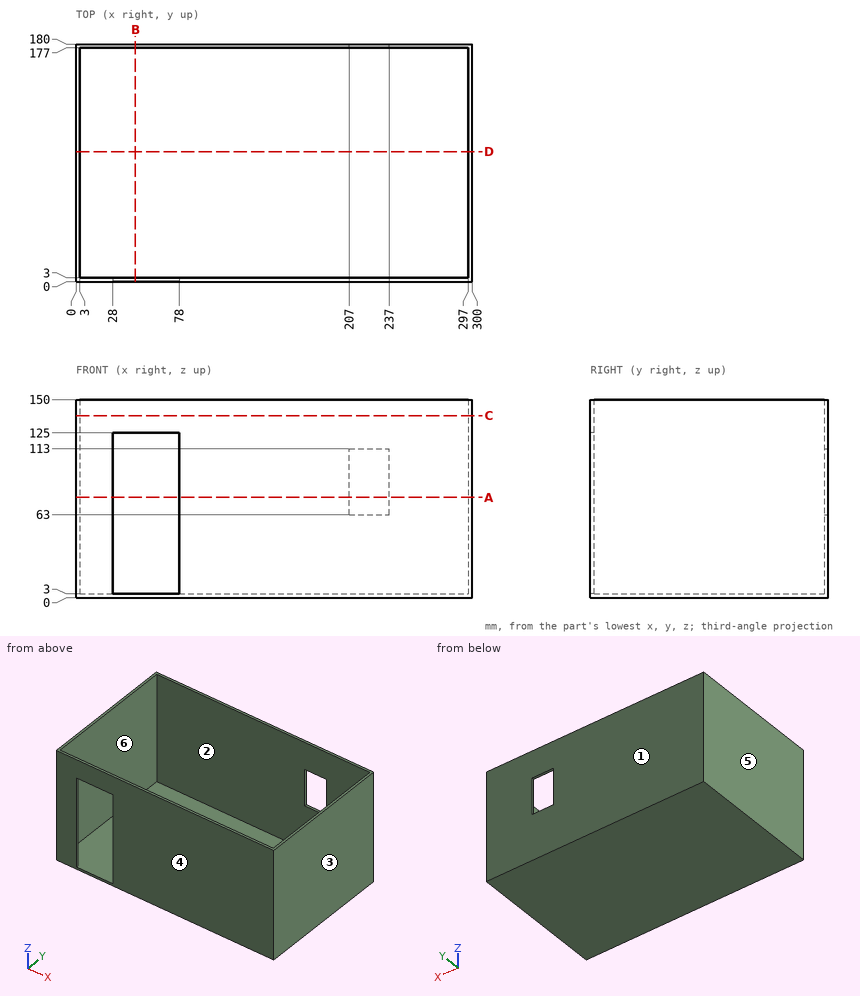
Could you check a few things on this drawing? It's one solid part, dimensions in mm from its lowest x, y, z. A direction names the side the tool comes from. Give positions to 0.01 mm unless a question says otherwise; leave off trailing zeros. Write each loop counter-clockwise with the first axis right and the second up, starting at its lowest first coordinate (ties: lowest second). Pieces come first, ordered by that corner, then holes. Notation, with made-up numbers: (16.25, 40) -> (73.25, 40) arc R27 cw to (73.25, 69) -> close; hole circle Ø6 at (66.25, 12.5). An arc over 180 degrees is marked (long way). Answer as a JSON object with one key per item and string values.
Q1. Suppose I cut it at A-A on z = 76. Write out the boundary of the cut face in (x, y), then the cut area to 3 significant figures.
Taken from the geometry:
{"outline": "(0, 0) -> (28, 0) -> (28, 3) -> (3, 3) -> (3, 177) -> (207, 177) -> (207, 180) -> (0, 180) -> close; (78, 0) -> (300, 0) -> (300, 180) -> (237, 180) -> (237, 177) -> (297, 177) -> (297, 3) -> (78, 3) -> close", "area": "2,600 mm²"}
Q2. Please list where these lines run through material, in increasing order: L1, parallel to X at y = 126.5, z = 97; L2, parallel to Y at x = 159.5, z = 60; L3, parallel to Z at x = 212, y = 39.
Taken from the geometry:
{"L1": "x = 0 to 3, 297 to 300", "L2": "y = 0 to 3, 177 to 180", "L3": "z = 0 to 3"}
Q3. Which directions (+Z, -Z, +X, -X, +Y, -Y) give clear straight access to the entire face, cutting with the end or side of a thin tool? Please do the marked faces 1 and 2.
Taken from the geometry:
{"face 1": "+Z, -Z, +X, -X, +Y", "face 2": "+Z"}
Q4. Suppose I cut it at D-D on y = 98.5. Write out the boundary of the cut face in (x, z), then the cut area to 3 significant figures.
Taken from the geometry:
{"outline": "(0, 0) -> (300, 0) -> (300, 150) -> (297, 150) -> (297, 3) -> (3, 3) -> (3, 150) -> (0, 150) -> close", "area": "1,780 mm²"}
Q5. Suppose I cut it at B-B on x = 45. Write out the boundary of the cut face in (y, z).
Taken from the geometry:
{"outline": "(0, 0) -> (180, 0) -> (180, 150) -> (177, 150) -> (177, 3) -> (0, 3) -> close; (0, 125) -> (3, 125) -> (3, 150) -> (0, 150) -> close"}
Q6. Will these pins go through, and if not, where does the flat tip stop? pin 1 Ø2.5 at (x, y) = (227.5, 179) entering from -Z; pin 2 Ø8 at (x, y) = (126, 44) entering from +Z.
Taken from the geometry:
{"pin 1": "stops at z = 0", "pin 2": "stops at z = 3"}
Q7. We'd pull the mould along X, two halves only. Please class the marked faces 3, 4, 5 and 6: released by +X, released by -X, zero draft, split by the parting line, or undercut.
Taken from the geometry:
{"face 3": "released by +X", "face 4": "zero draft", "face 5": "released by -X", "face 6": "undercut"}
Q8. Suppose I cut it at C-C on z = 138. Write out the boundary of the cut face in (x, y), then the cut area to 3 significant figures.
Taken from the geometry:
{"outline": "(0, 0) -> (300, 0) -> (300, 180) -> (0, 180) -> close; hole (3, 3) -> (297, 3) -> (297, 177) -> (3, 177) -> close", "area": "2,840 mm²"}
